Can you work these out from the model? Positions are in its coordinate system, mm. A direction names the side the tool comes from. Round coordinates to 2 decimals unless told otherwise and drop trailing zeros. Order: outer loops, then holes, each group sorted by start corner. A loop starts at its lowest first (then second) coordinate and runs counter-clockwise, first axis right, second up. Notation, with made-up numbers: (14.5, 14.5) -> (25.5, 14.5) arc R11 cw to (25.5, 20.5) -> close; hole circle Ø8 at (-29.5, 69). An arc over 180 degrees is marked (long way). Use a Markdown table: item, result. Add a question column.
Q1. If we section it at C-C on y = 6: List the corners of the cut face in (x, z) for me, plus the area to 3 significant figures.
Q2. I need wall thicknesses on line 1 along X through (y, z) = (3.25, -2.75); line 2 along X through (y, z) = (2.75, -3.25); line 3 along Z through (x, y) = (-6, 4.25). Which ranges of each line are inside material? Lowest first, please. Write a range as [from, to].
Q3. If we section it at A-A on x = -6: List the corners of the cut face in (y, z) for me.
Q4. For faces 1 (the face through (-5, 2, -4.746)), 2 (the face through (-10, 6.223, -5)), 3 (the face through (-14.036, 2.866, -5.403)), which set-ups out of +Z, -Z, +X, -X, +Y, -Y let a thin tool reach every point of the face, with its end or its side?
Q5. I'm going to push flat-ended pins straight in: pin 1 Ø2.5 at (x, y) = (-3.175, 3.175) entering from -Z; pin 2 Ø1.9 at (x, y) = (-4, 3) entering from +Z; pin 3 Ø0.6 at (x, z) = (-10, -5) entering from +Y. Where does each tip first touch, or does it pass through?
Q6. We'd pull the mould along Y, two halves only. Please class faces 4 (the face through (-7, 6.35, -4)), 5 (the face through (-7, 0, -4)), 6 (the face through (-7.958, 3.131, -4.984)), 7 (the face through (-3.745, 1.364, -2.406)): +Y half, -Y half, draft (parallel to the pull), parting line (faces both ways), or undercut.
Q7. If we section it at D-D on y = 1.5: List the corners of the cut face in (x, z) for me, plus the area to 3 significant figures.
Autodesk Inventor part; units mm, degrees
ref_plane "YZ Plane" through (0, 0, 0) normal (1, 0, 0) x (0, 1, 0)
ref_plane "XZ Plane" through (0, 0, 0) normal (0, 1, 0) x (-1, 0, 0)
ref_plane "XY Plane" through (0, 0, 0) normal (0, 0, 1) x (1, 0, 0)
sketch "Sketch1" plane through (0, 0, 0) normal (0, 1, 0) x (-1, 0, 0)
  line L0 (0, 0) -> (15, 0)
  line L1 (15, 0) -> (15, -10)
  line L2 (15, -10) -> (0, -10)
  line L3 (0, -10) -> (0, 0)
  line L4 (0, -5) -> (7.5006, -5)
  circle A0 centre (7.5006, -5) radius 0.4572
  line L5 (0, -5.254) -> (7.1205, -5.254)
  line L6 (0, -4.746) -> (7.1205, -4.746)
  dimension "d0" = 15
  dimension "d1" = 10
  dimension "d2" = 7.5006
  dimension "d3" = 0.9144
  dimension "d4" = 0.254
  dimension "d5" = 0.254
extrude "Extrusion1" add sketch "Sketch1" along normal blind 6.35 contours L0 L1 L2 L3 L5 A0 L6
sketch "Sketch2" plane through (-15, 0, 0) normal (0, 0, 1) x (1, 0, 0)
  line L0 (7.8795, 0) -> (15, 0)
  line L1 (15, 0) -> (8.65, 6.35)
  line L2 (15, 6.35) -> (7.8795, 6.35)
  line L3 (15, 0) -> (23.9803, 0) construction
  circle A0 centre (11.825, 3.175) radius 1.7526
  line L4 (15, 0) -> (0, 0)
  line L5 (0, 0) -> (6.35, 6.35)
  line L6 (7.0422, 6.35) -> (7.8795, 6.35)
  line L7 (0, 0) -> (8.9803, 0) construction
  circle A1 centre (3.175, 3.175) radius 1.7526
  dimension "d8" = 135
  dimension "d9" = 3.5052
  dimension "d10" = 45
  dimension "d11" = 3.5052
sketch "Sketch3" plane through (-15, 0, -10) normal (-1, 0, 0) x (0, 0, 1)
  line L0 (0, 6.35) -> (10, 6.35)
  line L1 (0, 6.35) -> (10, 0)
  circle A0 centre (5, 3.175) radius 0.508
  dimension "d30" = 1.016
extrude "Extrusion2" cut sketch "Sketch3" against normal blind 3.5001
hole "Hole3" at (-11.825, 3.175, 0) direction (0, 0, -1) diameter 2.6416 end through all
sketch "Sketch4" plane through (0, 0, -10) normal (0, 0, -1) x (-1, 0, 0)
  line L0 (0, 0) -> (6.35, 6.35)
  line L1 (7.1205, 6.35) -> (0, 6.35)
  line L2 (0, 0) -> (8.9803, 0) construction
  line L3 (6.35, 6.35) -> (3.175, 3.175)
  circle A0 centre (3.175, 3.175) radius 1.3208
  dimension "d44" = 45
  dimension "d45" = 2.6416
hole "Hole4" at (-3.175, 3.175, -10) direction (0, 0, 1) diameter 2.6416 depth 5 tip angle 118
hole "Hole5" at (-3.175, 3.175, 0) direction (0, 0, -1) diameter 3.7973 depth 5 tip angle 118
sketch "Sketch5" plane through (0, 6.35, 0) normal (0, 1, 0) x (1, 0, 0)
  arc A0 (-7.1205, 5.254) -> (-7.1205, 4.746) centre (-7.5006, 5) ccw
  circle A1 centre (-7.5006, 5) radius 3.81
  circle A2 centre (-7.5006, 5) radius 16.51
  line L0 (-15, 10) -> (-15, 0)
  line L1 (-15, 0) -> (-8.65, 0)
  line L2 (-8.65, 0) -> (-8.65, -6.35)
  line L3 (-8.65, -6.35) -> (-15, -6.35)
  line L4 (-15, -6.35) -> (-15, 0)
  line L5 (-15, 10) -> (-8.65, 10)
  line L6 (-8.65, 10) -> (-8.65, 16.35)
  line L7 (-8.65, 16.35) -> (-15, 16.35)
  line L8 (-15, 16.35) -> (-15, 10)
  circle A3 centre (-7.5006, 5) radius 18.4277
  line L9 (-11.825, -9.8552) -> (-14.6952, -9.8552)
  line L10 (-14.6952, -9.8552) -> (-14.6952, -6.35)
  line L11 (-11.825, -9.8552) -> (-8.9548, -9.8552)
  line L12 (-8.9548, -9.8552) -> (-8.9548, -6.35)
  point P0 (0, 0)
  dimension "d60" = 7.62
  dimension "d61" = 33.02
  dimension "d62" = 6.35
  dimension "d63" = 6.35
  dimension "d64" = 6.35
  dimension "d65" = 6.35
  dimension "d66" = 36.8554
  dimension "d68" = 2.8702
  dimension "d69" = 2.8702
sketch "Sketch6" plane through (0, 6.35, 0) normal (0, 1, 0) x (1, 0, 0)
  arc A0 (-7.1205, 5.254) -> (-7.1205, 4.746) centre (-7.5006, 5) ccw
  line L0 (-7.9578, 5) -> (-8.8722, 5)
  line L1 (-8.8722, 5) -> (-8.8722, 5.9957)
  line L2 (-8.8722, 5.9957) -> (-11.1735, 5.9957)
  line L3 (-11.1735, 5.9957) -> (-11.1735, 4.0043)
  line L4 (-11.1735, 4.0043) -> (-8.8722, 4.0043)
  line L5 (-8.8722, 4.0043) -> (-8.8722, 5.9957)
  line L6 (-11.1735, 5.9957) -> (-21.1734, 5.9957)
  point P0 (0, 0)
  dimension "d70" = 0.9144
  dimension "d79" = 0.9957
  dimension "d80" = 2.3012
  dimension "d81" = 1.9914
  dimension "d84" = 10
extrude "Extrusion4" cut sketch "Sketch6" against normal blind 0.127
properties part number "clamp(6-32)-th"
Answer below:
| question | item | result |
|---|---|---|
| 1 | outline | (-15, -10) -> (0, -10) -> (0, -5.25) -> (-7.12, -5.25) arc R0.46 cw (long way) to (-7.12, -4.75) -> (0, -4.75) -> (0, 0) -> (-15, 0) -> close |
| 1 | area | 146 mm² |
| 2 | line 1 | [-15, -13.14], [-10.51, -5.07], [-1.28, 0] |
| 2 | line 2 | [-15, -13.08], [-10.57, -5.03], [-1.32, 0] |
| 2 | line 3 | [-10, -5.25], [-4.75, 0] |
| 3 | outline | (0, -10) -> (6.35, -10) -> (6.35, -5.25) -> (0, -5.25) -> close; (0, -4.75) -> (6.35, -4.75) -> (6.35, 0) -> (0, 0) -> close |
| 4 | face 1 | +X, +Y, -Y |
| 4 | face 2 | +Y |
| 4 | face 3 | -X |
| 5 | pin 1 | through |
| 5 | pin 2 | z = -5.25 |
| 5 | pin 3 | y = 6.22 |
| 6 | face 4 | +Y half |
| 6 | face 5 | -Y half |
| 6 | face 6 | draft |
| 6 | face 7 | undercut |
| 7 | outline | (-15, -10) -> (0, -10) -> (0, -5.25) -> (-7.12, -5.25) arc R0.46 cw (long way) to (-7.12, -4.75) -> (-4.07, -4.75) -> (-4.07, 0) -> (-15, 0) -> close; (-2.28, -4.75) -> (0, -4.75) -> (0, 0) -> (-2.28, 0) -> close |
| 7 | area | 137 mm² |
